Verification items for this drawing (mm, ordinates from the low corner). A direction names the side the tool comes from. Give positions to 0.01 mm unless a question says otherwise; leave off trailing zeros. Order: outer loops, then holes, each group sorted by start corner. A loop starts at its lowest first (then second) coordinate and runs counter-clockwise, first axis right, second up. Notation, with made-up numbers: M 78.5,-34 L 126.5,-34 A18 cw 126.5,-13 Z; hole C 33.25,-12 d7. An arc over 180 degrees is marked long. Answer as a JSON object with one key per item and string values.
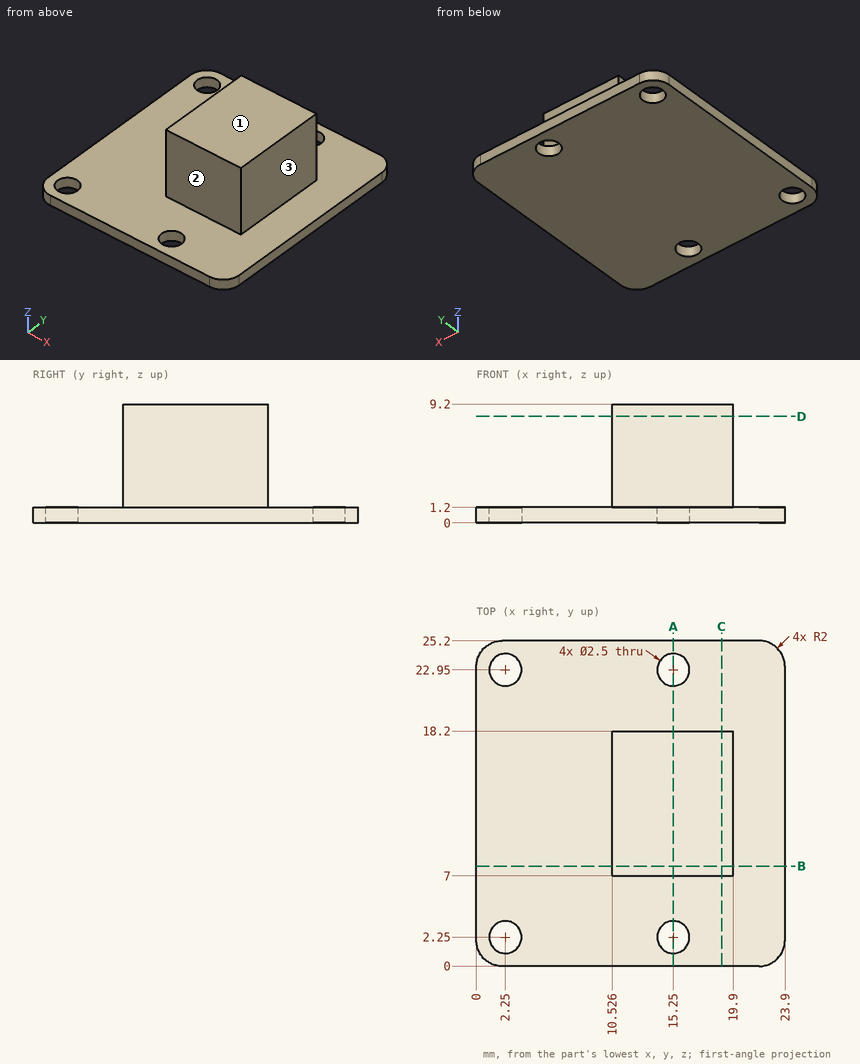
Q1. Tool access check on the marked faces 1, 2 and 3. Record the directions out of +Z, -Z, +X, -X, +Y, -Y that give a thin tool (end or side, any length) a straight path to the whole face; none if there is none.
Resolved:
{"face 1": "+Z, +X, -X, +Y, -Y", "face 2": "+Z, +X, -X, -Y", "face 3": "+Z, +X, +Y, -Y"}
Q2. Section check C-C on x = 19. Record the cut outline in (y, z).
Resolved:
{"outline": "M 0,0 L 25.2,0 L 25.2,1.2 L 18.2,1.2 L 18.2,9.2 L 7,9.2 L 7,1.2 L 0,1.2 Z"}
Q3. Section check D-D on z = 8.25. Record the cut outline in (x, y), then the cut area to 3 significant figures.
Resolved:
{"outline": "M 10.53,7 L 19.9,7 L 19.9,18.2 L 10.53,18.2 Z", "area": "105 mm²"}
Q4. Section check B-B on y = 7.75. Record the cut outline in (x, z), then the cut area to 3 significant figures.
Resolved:
{"outline": "M 0,0 L 23.9,0 L 23.9,1.2 L 19.9,1.2 L 19.9,9.2 L 10.53,9.2 L 10.53,1.2 L 0,1.2 Z", "area": "104 mm²"}
Q5. Material ranges on L1, parallel to Y at x = 15.25, z = 0.9; L2, parallel to X at y = 9.75, z = 6.25; L3, parallel to Z at x = 15.75, y = 5.75, recorded low to high.
Resolved:
{"L1": "y = 0 to 1, 3.5 to 21.7, 24.2 to 25.2", "L2": "x = 10.53 to 19.9", "L3": "z = 0 to 1.2"}
Q6. Gauge pin test, flat ends, axial feed: pin 1 Ø2 at (x, y) = (15.25, 22.95) entering from +Z; pin 2 Ø2 at (y, z) = (12.5, 1) entering from -X; pin 3 Ø4 at (x, z) = (14, 7) entering from +Y; pin 4 Ø2 at (x, y) = (5.5, 3) entering from +Z. Record the tip position at first contact, or that the pin passes through.
Resolved:
{"pin 1": "passes through", "pin 2": "stops at x = 0", "pin 3": "stops at y = 18.2", "pin 4": "stops at z = 1.2"}
Q7. Section check A-A on x = 15.25. Record the cut outline in (y, z).
Resolved:
{"outline": "M 0,0 L 1,0 L 1,1.2 L 0,1.2 Z; M 3.5,0 L 21.7,0 L 21.7,1.2 L 18.2,1.2 L 18.2,9.2 L 7,9.2 L 7,1.2 L 3.5,1.2 Z; M 24.2,0 L 25.2,0 L 25.2,1.2 L 24.2,1.2 Z"}
